Geometry: see drawing. Coordinates: mm, zero at the bounding-box minimum. A direction names the side the tool comes from. Give positions to 0.01 mm unless a question says otherwise; leave off trailing zeros. Loops run counter-clockwise (first coordinate to the right, second up) from the corner with the lowest first, then second, coordinate; pieces in that order, holes last. Notation, with made-up numbers: M 52,59 L 57,59 A13 cw 57,72 Z; hole C 3.25,78.25 d4. An arc over 180 degrees is marked long. Answer in a Markdown table with one row per item.
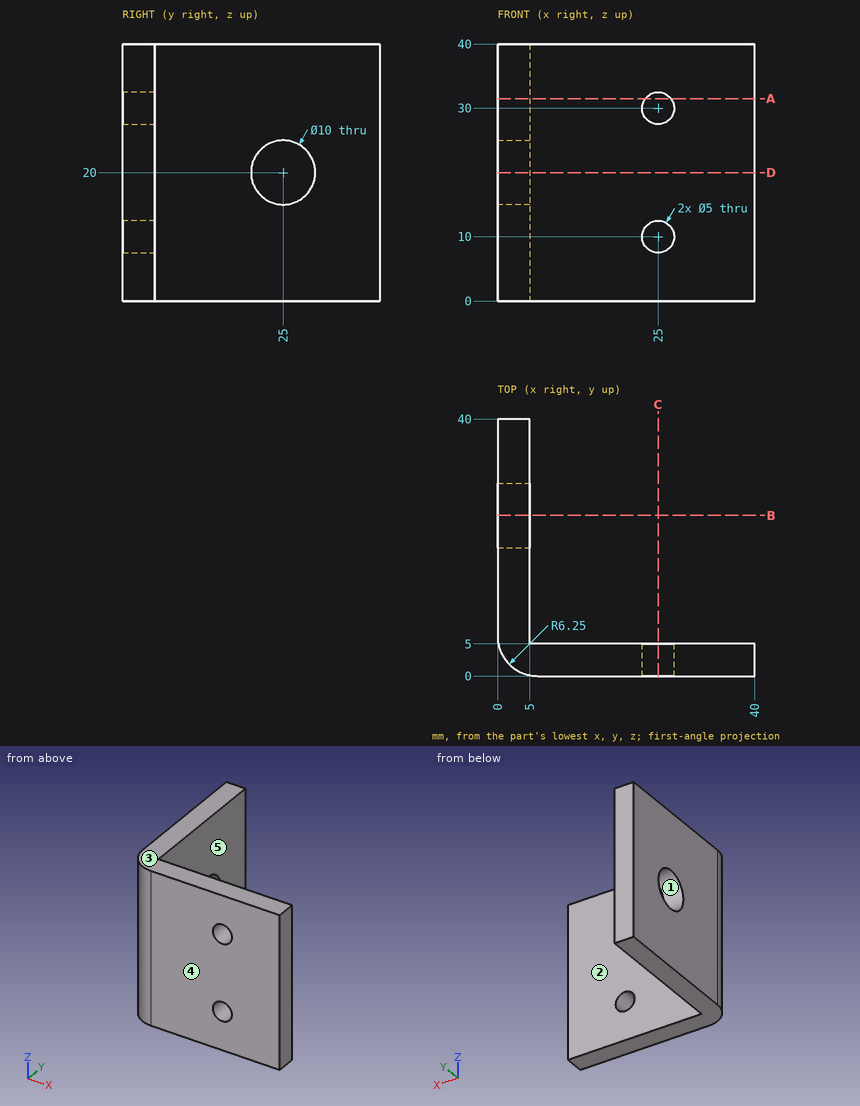
1) Section C-C, the plane x = 25. Return loops of the section in (y, z).
Reply:
| item | result |
|---|---|
| outline | M 0,0 L 5,0 L 5,7.5 L 0,7.5 Z; M 0,12.5 L 5,12.5 L 5,27.5 L 0,27.5 Z; M 0,32.5 L 5,32.5 L 5,40 L 0,40 Z |
2) Section A-A, the plane z = 31.5. Return loops of the section in (x, y), then the cut area to 3 significant figures.
Reply:
| item | result |
|---|---|
| outline | M 0,6.25 A6.25 ccw 6.25,0 L 23,0 L 23,5 L 5,5 L 5,40 L 0,40 Z; M 27,0 L 40,0 L 40,5 L 27,5 Z |
| area | 347 mm² |
3) Section B-B, the plane y = 25. Return loops of the section in (x, z), then the cut area to 3 significant figures.
Reply:
| item | result |
|---|---|
| outline | M 0,0 L 5,0 L 5,15 L 0,15 Z; M 0,25 L 5,25 L 5,40 L 0,40 Z |
| area | 150 mm² |
4) Section D-D, the plane z = 20. Return loops of the section in (x, y), then the cut area to 3 significant figures.
Reply:
| item | result |
|---|---|
| outline | M 0,6.25 A6.25 ccw 6.25,0 L 40,0 L 40,5 L 5,5 L 5,20 L 0,20 Z; M 0,30 L 5,30 L 5,40 L 0,40 Z |
| area | 317 mm² |
5) Material intervals for L1, parallel to X at y = 17, z = 24; L2, parallel to X at y = 3, z = 31.5, sorted ascending.
Reply:
| item | result |
|---|---|
| L1 | x = 0 to 5 |
| L2 | x = 0.91 to 23, 27 to 40 |
6) Pull-direction query (Z, two-part tool) for the marked faces 1, 2 and 3; classes: released by +Z, released by -Z, zero draft, split by the parting line, or undercut.
Reply:
| item | result |
|---|---|
| face 1 | undercut |
| face 2 | zero draft |
| face 3 | released by +Z |
7) Set-up query: the marked faces 4 and 5. Return all of +Z, -Z, +X, -X, +Y, -Y with unobstructed straight access to the full face (end or side cutting, diameter ignored); none if empty.
Reply:
| item | result |
|---|---|
| face 4 | +Z, -Z, +X, -X, -Y |
| face 5 | +Z, -Z, +X, +Y |
8) Pin query (flat end, axial travel): pin 1 Ø4 at (y, z) = (32, 29) entering from +X; pin 2 Ø8 at (x, z) = (25, 10) entering from +Y; pin 3 Ø8 at (x, y) = (8, 16.5) entering from +Z. Return the tip coordinate at first contact, or that it passes through.
Reply:
| item | result |
|---|---|
| pin 1 | stops at x = 5 |
| pin 2 | stops at y = 5 |
| pin 3 | stops at z = 40 |
